Part model, mm, in its own coordinate system. Give positions to 0.01 mm unless a question says otherwise; leave off trailing zeros. Answer as a JSON object with one key per item and string values.
from build123d import *

# Parameters (mm, degrees)
SALIENTE_EXTRUIR1_DEPTH = 652
CORTAR_EXTRUIR1_DEPTH   = 653
CORTAR_EXTRUIR2_DEPTH   = 653
CORTAR_EXTRUIR3_DEPTH   = 653
CORTAR_EXTRUIR4_DEPTH   = 653
CORTAR_EXTRUIR5_DEPTH   = 653
CORTAR_EXTRUIR6_DEPTH   = 653
CORTAR_EXTRUIR7_DEPTH   = 0.002166667
CORTAR_EXTRUIR8_DEPTH   = 0.002166667
CORTAR_EXTRUIR9_DEPTH   = 0.002166667
CORTAR_EXTRUIR10_DEPTH  = 0.002166667
NGULO_DE_SALIDA1_ANGLE  = 45.1469538
CHAFL_N1_SIZE           = 0.4
REDONDEO1_R             = 0.130000023
MATRIZL2_COUNT          = 32
MATRIZL2_PITCH          = 20


with BuildPart() as part:
    # Croquis1 → Saliente-Extruir1 (new body)
    with BuildSketch(Plane.XZ):
        Polygon((4.5, 0), (4.5, 6.01167813), (4.1, 6.50000002), (-4.1, 6.50000002), (-4.5, 6.01167813), (-4.5, 0), align=None)
    extrude(amount=-SALIENTE_EXTRUIR1_DEPTH)

    # Croquis2 → Cortar-Extruir1 (cut, through all)
    with BuildSketch(Plane(origin=(0, 652, 0), x_dir=(-1, 0, 0), z_dir=(0, 1, 0))):
        with BuildLine():
            Line((-4.5, 4.88017535), (-4.5, 4.03150278))
            Line((-4.5, 4.03150278), (-3.819258765, 4.03150278))
            ThreePointArc((-3.819258765, 4.03150278), (-3.21946318, 4.455839065), (-3.819258765, 4.88017535))
            Line((-3.819258765, 4.88017535), (-4.5, 4.88017535))
        make_face()
    extrude(amount=-CORTAR_EXTRUIR1_DEPTH, mode=Mode.SUBTRACT)

    # Croquis3 → Cortar-Extruir2 (cut, through all)
    with BuildSketch(Plane(origin=(0, 652, 0), x_dir=(-1, 0, 0), z_dir=(0, 1, 0))):
        with BuildLine():
            Line((-4.026513856, 4.03150278), (-4.5, 4.03150278))
            Line((-4.5, 4.03150278), (-4.5, 3.583620931))
            ThreePointArc((-4.5, 3.583620931), (-4.223645982, 3.76568645), (-4.026513856, 4.03150278))
        make_face()
    extrude(amount=-CORTAR_EXTRUIR2_DEPTH, mode=Mode.SUBTRACT)

    # Croquis4 → Cortar-Extruir3 (cut, through all)
    with BuildSketch(Plane(origin=(0, 652, 0), x_dir=(-1, 0, 0), z_dir=(0, 1, 0))):
        with BuildLine():
            Line((-4.5, 5.328056964), (-4.5, 4.88017535))
            Line((-4.5, 4.88017535), (-4.026513974, 4.88017535))
            ThreePointArc((-4.026513974, 4.88017535), (-4.223646078, 5.145991535), (-4.5, 5.328056964))
        make_face()
    extrude(amount=-CORTAR_EXTRUIR3_DEPTH, mode=Mode.SUBTRACT)

    # Croquis5 → Cortar-Extruir4 (cut, through all)
    with BuildSketch(Plane(origin=(0, 652, 0), x_dir=(-1, 0, 0), z_dir=(0, 1, 0))):
        with BuildLine():
            Line((4.5, 4.03150278), (4.5, 4.88017535))
            Line((4.5, 4.88017535), (3.819258765, 4.88017535))
            ThreePointArc((3.819258765, 4.88017535), (3.21946318, 4.455839065), (3.819258765, 4.03150278))
            Line((3.819258765, 4.03150278), (4.5, 4.03150278))
        make_face()
    extrude(amount=-CORTAR_EXTRUIR4_DEPTH, mode=Mode.SUBTRACT)

    # Croquis6 → Cortar-Extruir5 (cut, through all)
    with BuildSketch(Plane(origin=(0, 652, 0), x_dir=(-1, 0, 0), z_dir=(0, 1, 0))):
        with BuildLine():
            Line((4.026513826, 4.88017535), (4.5, 4.88017535))
            Line((4.5, 4.88017535), (4.5, 5.328057255))
            ThreePointArc((4.5, 5.328057255), (4.223645966, 5.145991706), (4.026513826, 4.88017535))
        make_face()
    extrude(amount=-CORTAR_EXTRUIR5_DEPTH, mode=Mode.SUBTRACT)

    # Croquis7 → Cortar-Extruir6 (cut, through all)
    with BuildSketch(Plane(origin=(0, 652, 0), x_dir=(-1, 0, 0), z_dir=(0, 1, 0))):
        with BuildLine():
            Line((4.5, 3.583620926), (4.5, 4.03150278))
            Line((4.5, 4.03150278), (4.026513851, 4.03150278))
            ThreePointArc((4.026513851, 4.03150278), (4.223645987, 3.765686455), (4.5, 3.583620926))
        make_face()
    extrude(amount=-CORTAR_EXTRUIR6_DEPTH, mode=Mode.SUBTRACT)

    # Croquis8 → Cortar-Extruir7 (cut)
    with BuildSketch(Plane(origin=(0, 652, 0), x_dir=(-1, 0, 0), z_dir=(0, 1, 0))):
        Polygon((0.891369267, 3.403698133), (0.714701433, 3.168235633), (0.2187042, 2.61105), (1.0945792, 2.61105), (1.0945792, 2.695983333), (0.398689633, 2.695983333), (0.794326433, 3.149466667), (0.9743123, 3.3891), (1.067110588, 3.573407857), (0.95413722, 3.802321701), (0.7876908, 3.88505), (0.54301, 3.88505), (0.375434678, 3.803592619), (0.295011167, 3.6384023), (0.295011167, 3.562), (0.3812718, 3.562), (0.3812718, 3.631766667), (0.437672733, 3.743620833), (0.549645633, 3.800116667), (0.7802262, 3.800116667), (0.893028067, 3.743810633), (0.976240026, 3.576039029), align=None)
    extrude(amount=-CORTAR_EXTRUIR7_DEPTH, mode=Mode.SUBTRACT)

    # Croquis9 → Cortar-Extruir8 (cut)
    with BuildSketch(Plane.XZ):
        Polygon((-0.214632167, 3.88505), (-0.953983333, 3.88505), (-0.953983333, 2.61105), (-0.214632167, 2.61105), (-0.214632167, 2.695983333), (-0.86905, 2.695983333), (-0.86905, 3.205583333), (-0.5123963, 3.205583333), (-0.5123963, 3.290516667), (-0.86905, 3.290516667), (-0.86905, 3.800116667), (-0.214632167, 3.800116667), align=None)
    extrude(amount=-CORTAR_EXTRUIR8_DEPTH, mode=Mode.SUBTRACT)

    # Croquis10 → Cortar-Extruir9 (cut)
    with BuildSketch(Plane(origin=(0, 652, 0), x_dir=(-1, 0, 0), z_dir=(0, 1, 0))):
        Polygon((-0.214632167, 3.88505), (-0.953983333, 3.88505), (-0.953983333, 2.61105), (-0.214632167, 2.61105), (-0.214632167, 2.695983333), (-0.86905, 2.695983333), (-0.86905, 3.205583333), (-0.5123963, 3.205583333), (-0.5123963, 3.290516667), (-0.86905, 3.290516667), (-0.86905, 3.800116667), (-0.214632167, 3.800116667), align=None)
    extrude(amount=-CORTAR_EXTRUIR9_DEPTH, mode=Mode.SUBTRACT)

    # Croquis11 → Cortar-Extruir10 (cut)
    with BuildSketch(Plane.XZ):
        Polygon((0.510057167, 3.620830633), (0.6071, 3.718655633), (0.6071, 2.609403333), (0.692033333, 2.609403333), (0.692033333, 3.883403333), (0.6741176, 3.883403333), (0.6741176, 3.795069794), (0.3690544, 3.640736667), (0.3690544, 3.551253333), align=None)
    extrude(amount=-CORTAR_EXTRUIR10_DEPTH, mode=Mode.SUBTRACT)

    # Ángulo de salida1
    ngulo_de_salida1_faces = [part.faces().sort_by_distance(p)[0] for p in [
        (0.6741176, 0.001083333, 3.839236564),
    ]]
    draft(ngulo_de_salida1_faces, Plane(origin=(0.692033333, 0.002166667, 3.883403333), x_dir=(-1, 0, 0), z_dir=(0, 0, -1)), NGULO_DE_SALIDA1_ANGLE)

    # Chaflán1
    chafl_n1_edges = [part.edges().sort_by_distance(p)[0] for p in [
        (-4.5, 326, 0),
        (4.5, 326, 0),
    ]]
    chamfer(chafl_n1_edges, length=CHAFL_N1_SIZE)

    # Redondeo1
    redondeo1_edges = [part.edges().sort_by_distance(p)[0] for p in [
        (4.026513856, 326, 4.03150278),
        (4.5, 326, 3.583620931),
        (4.5, 326, 5.328056964),
        (4.026513974, 326, 4.88017535),
        (-4.026513826, 326, 4.88017535),
        (-4.5, 326, 5.328057255),
        (-4.5, 326, 3.583620926),
        (-4.026513851, 326, 4.03150278),
    ]]
    fillet(redondeo1_edges, radius=REDONDEO1_R)

    # Croquis34 → Taladro roscado M3.5x0.61 (revolve, cut)
    with BuildSketch(Plane(origin=(0, 16, 0), x_dir=(0, 1, 0), z_dir=(1, 0, 0))):
        Polygon((0, 0), (0, 8), (3, 8), (3, 3), (1.5, 3), (1.5, 0), align=None)
    taladro_roscado_m3_5x0_61 = revolve(axis=Axis((0, 16, -6.35), (0, 0, 1)), mode=Mode.SUBTRACT)

    # MatrizL2: Taladro roscado M3.5x0.61 ×32
    with Locations(*[(0, i * MATRIZL2_PITCH, 0) for i in range(1, MATRIZL2_COUNT)]):
        add(taladro_roscado_m3_5x0_61, mode=Mode.SUBTRACT)


solid = part.part
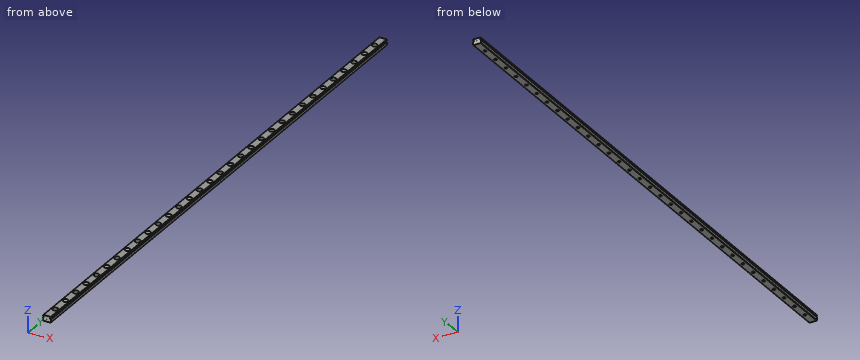
1. Cut at A-A on z = 1.5. State how many separate pieces and enclosed holes the cut face has, plus the area to 3 significant figures.
Worked answers:
{"separate pieces": "1", "enclosed holes": "32", "area": "5,640 mm^2"}
2. Pin check, flat tips, straight feed: P1, Ø3, axis at x = 1, y = 136, coming from the +Z side; P2, Ø1, axis at y = 154.5, z = 4.5, coming from the -X side. Stop position of each tip, or through.
Worked answers:
{"P1": "stops at z = 3", "P2": "stops at x = -4.1"}
3. Probe line 1 along X through (y, z) = (36, 1.8); line 2 along Z through (x, y) = (-3.5, 244.5); line 3 along X through (y, z) = (456, 5.45). List the from-to ranges inside material, lowest first.
Worked answers:
{"line 1": "x = -4.5 to -1.5, 1.5 to 4.5", "line 2": "z = 0 to 4.04, 4.87 to 6.5", "line 3": "x = -4.5 to -3, 3 to 4.5"}
